Autodesk Inventor part; units mm, degrees
ref_plane "YZ Plane" through (0, 0, 0) normal (1, 0, 0) x (0, 1, 0)
ref_plane "XZ Plane" through (0, 0, 0) normal (0, 1, 0) x (-1, 0, 0)
ref_plane "XY Plane" through (0, 0, 0) normal (0, 0, 1) x (1, 0, 0)
sketch "Sketch1" plane through (0, 0, 0) normal (0, 0, 1) x (1, 0, 0)
  line L0 (0, 0) -> (0, 3)
  line L1 (0, 3) -> (15, 3)
  line L2 (15, 3) -> (15, 4)
  line L3 (15, 4) -> (30, 4)
  line L4 (30, 4) -> (30, 0)
  line L5 (30, 0) -> (0, 0)
  line L6 (29.5, 0) -> (29.5, 2)
  line L7 (29.5, 2) -> (30, 2)
  line L8 (29.5, 1.15) -> (27, 1.15)
  line L9 (27, 1.15) -> (26.2814, 0)
  line L10 (26.2814, 0) -> (29.5, 0)
  point P0 (0, 1.5)
  point P1 (30, 2)
  dimension "d0" = 3
  dimension "d1" = 4
  dimension "d2" = 15
  dimension "d3" = 30
  dimension "d4" = 2
  dimension "d5" = 0.5
  dimension "d27" = 1.15
  dimension "d28" = 58
  dimension "d29" = 2.5
revolve "Revolution1" add sketch "Sketch1" angle 360 about axis through (30, 0, 0) along (-1, 0, 0) contours L0 L1 L2 L3 L4 L7 L6 L8 L9 L5
chamfer "Chamfer1" distance 0.5 angle 45 2 edges at (0, -3, 0) (15, -4, 0)
chamfer "Chamfer2" distance 0.1 angle 45 1 edges at (30, -4, 0)
sketch "Sketch2" plane through (0, 0, 0) normal (0, 1, 0) x (-1, 0, 0)
  circle A0 centre (-28, 0) radius 0.8
  line L0 (-30, -2) -> (-30, 2)
  point P0 (0, 0)
  dimension "d13" = 1.6
  dimension "d14" = 2
extrude "Extrusion1" cut sketch "Sketch2" along normal mid plane 10
chamfer "Chamfer4" distance 0.2 angle 45 3 edges at (28, 3.9192, 0.8) (28.0001, 3.9192, -0.8) (28.8, -4, -0.0013)
thread "Thread2"
thread "Thread3"
properties part number "Sp mu SM holder"
The listing builds one solid part. Answer for the finished solid, in the listing's coordinates (mm). A direction names the side the tool comes from. Round coordinates to 2 decimals unless told otherwise and drop trailing zeros. Order: outer loops, then holes, each group sorted by start corner. A loop starts at its lowest first (then second) coordinate and runs counter-clockwise, first axis right, second up. Notation, with made-up numbers: (71, -8) - (128, -8) arc R25 ccw to (128, 25) - close; hole circle Ø5 at (-1, 89). An arc over 180 degrees is marked (long way). Write item = value, one per line. Start each with the question number.
1) For faces 4 (the cylindrical face through (28.23, -0.15, -1.14)), 5 (the cylindrical face through (27.237, -2.292, 0.24)), 6 (the flat face through (15, 3, -1)), determine the directions among +Z, -Z, +X, -X, +Y, -Y from which every point of the face is accessible in a straight line to the end or side of a thin tool.
2) Given pin 1 (2 mm diameter, centred on y = 0.5, z = 1.5, fed in from +X), flat-ended and moving along its own axis, determine where the tip first touches the part or whether it passes through.
3) For a pull along Y with two mould halves and no side action, classify faces 1 (the cylindrical face through (8, -3, 0)), 2 (the cylindrical face through (27.237, 2.292, -0.24)), 3 (the cylindrical face through (29.754, -0.434, -1.952)) as released by +Y, released by -Y, zero draft, split by the parting line, or undercut.
4) Straight lines are drawn through the part: L1, parallel to X at y = -2.25, z = 0; L2, parallel to X at y = 3.25, z = 0; L3, parallel to Z at x = 29.7, y = 0. For each, find the intervals that lie inside material, in ascending order.
5) Section B-B, the plane z = -0.5 is taken. Count the separate pieces of the cut face and the enclosed holes in it, plus the area to 3 significant figures.
6) Section C-C, the plane x = 20 is taken. Write down the section's boundary in (y, z).
7) Section A-A, the plane x = 8.5 is taken. Write down the section's boundary in (y, z).
Results list:
q1.face_4 = +X
q1.face_5 = +Y, -Y
q1.face_6 = -X
q2.pin_1 = 30
q3.face_1 = split by the parting line
q3.face_2 = zero draft
q3.face_3 = undercut
q4.L1 = 0 to 27.2, 28.8 to 30
q4.L2 = 15 to 27.2, 28.8 to 30
q4.L3 = -4 to -2, 2 to 4
q5.separate_pieces = 3
q5.enclosed_holes = 0
q5.area = 192 mm^2
q6.outline = circle Ø8 at (0, 0)
q7.outline = circle Ø6 at (0, 0)
